```python
from build123d import *

# Parameters (mm, degrees)
F1_DEPTH = 5
F2_R     = 5
F2_R_2   = 2.5
F3_DEPTH = 5
F4_R     = 1.5
F5_DEPTH = 5


with BuildPart() as f1:
    # F0 (on Front) → F1 (new body)
    with BuildSketch(Plane.XZ):
        with BuildLine():
            ThreePointArc((0, 43.75), (-17.67767, 36.42767), (-25, 18.75))
            Line((-25, 18.75), (-25, -18.75))
            ThreePointArc((-25, -18.75), (-17.67767, -36.42767), (0, -43.75))
            Line((0, -43.75), (37.5, -43.75))
            ThreePointArc((37.5, -43.75), (55.17767, -36.42767), (62.5, -18.75))
            Line((62.5, -18.75), (62.5, 18.75))
            ThreePointArc((62.5, 18.75), (55.17767, 36.42767), (37.5, 43.75))
            Line((37.5, 43.75), (0, 43.75))
        make_face()
    extrude(amount=F1_DEPTH)

    # F2 (on face) → F3 (join)
    with BuildSketch(Plane.XZ.offset(5)):
        with Locations((0, 18.75)):
            Circle(F2_R)
        with Locations((0, -18.75)):
            Circle(F2_R)
        with Locations((15, -31.978757)):
            Circle(F2_R_2)
    extrude(amount=F3_DEPTH)

    # F4 (on face) → F5 (join)
    with BuildSketch(Plane.XZ.offset(5)):
        with Locations((30, 18.75)):
            Circle(F4_R)
    extrude(amount=F5_DEPTH)


solid = f1.part
```
Geometry: final body of the model. Coordinates: model frame, mm. A direction names the side the tool comes from. Coordinates: 2 decimals unless noted, no trailing zeros. Loops run counter-clockwise (first coordinate to the right, second up) from the corner with the lowest first, then second, coordinate; pieces in that order, holes last. Notation, with made-up numbers: (-6, 35.5) -> (16, 35.5) arc R27 ccw to (16, 66.5) -> close; hole circle Ø11 at (-39.75, 42). An arc over 180 degrees is marked (long way). Use a Markdown table: item, result. Add a question column.
(1) Line query: line 1 along Y through (x, z) = (56, 0.5); line 2 along X through (y, z) = (-1.5, -19.5); line 3 along X through (y, z) = (-0.5, -39). Output: solid intervals per line, ascending.
(2) Section query A-A, the plane x = 30. Return loops of the section in (y, z), plus the area to 4 significant figures.
(3) Pin query (flat end, axial travel): pin 1 Ø3 at (y, z) = (-8.5, -30) entering from +X; pin 2 Ø1.5 at (y, z) = (-6.5, -10) entering from +X; pin 3 Ø1 at (x, z) = (-7.5, -24.5) entering from -Y. Return the tip coordinate at first contact, or that it passes through.
(4) Section query C-C, the plane z = 11. Return loops of the section in (x, y), plus the area to 4 significant figures.
(5) Access query for faces 1 (the cylindrical face through (54.982, -2.465, -36.621)), 2 (the cylindrical face through (14.67, -7.46, -29.5)). Directions: +Z, -Z, +X, -X, +Y, -Y. A direction counts if a zero-diameter tool reaches every point of the face in a straight line with its end or side. Return the directions, or none.
(6) Section query D-D, the plane x = 21. Return loops of the section in (y, z).
(7) Section query B-B, the plane y = -3.25. Return loops of the section in (x, z).
(8) Mould query, pull axis X, two halves, no side actions, for faces 3 (the cylindrical face through (-1.08, -7.46, -23.63)), 4 (the cylindrical face through (-17.9, -2.5, -36.2)), 5 (the cylindrical face through (28.89, -7.46, 19.76)), 6 (the flat face through (18, 0, 1)). Classes: pulls with the +X half, pulls with the -X half, needs draft (parallel to the pull), parting line crosses it, or undercut.
Answer:
| question | item | result |
|---|---|---|
| 1 | line 1 | y = -5 to 0 |
| 1 | line 2 | x = -24.99 to 62.49 |
| 1 | line 3 | x = -14.66 to 52.16 |
| 2 | outline | (-10, 17.25) -> (-5, 17.25) -> (-5, -43.75) -> (0, -43.75) -> (0, 43.75) -> (-5, 43.75) -> (-5, 20.25) -> (-10, 20.25) -> close |
| 2 | area | 452.5 mm^2 |
| 3 | pin 1 | stops at x = 17.45 |
| 3 | pin 2 | passes through |
| 3 | pin 3 | stops at y = -5 |
| 4 | outline | (-25, -5) -> (62.5, -5) -> (62.5, 0) -> (-25, 0) -> close |
| 4 | area | 437.5 mm^2 |
| 5 | face 1 | -Z, +X, +Y, -Y |
| 5 | face 2 | -Y |
| 6 | outline | (-5, -43.75) -> (0, -43.75) -> (0, 43.75) -> (-5, 43.75) -> close |
| 7 | outline | (-25, -18.75) arc R25 ccw to (0, -43.75) -> (37.5, -43.75) arc R25 ccw to (62.5, -18.75) -> (62.5, 18.75) arc R25 ccw to (37.5, 43.75) -> (0, 43.75) arc R25 ccw to (-25, 18.75) -> close |
| 8 | face 3 | parting line crosses it |
| 8 | face 4 | pulls with the -X half |
| 8 | face 5 | undercut |
| 8 | face 6 | needs draft |
